Check sheet for the drawn part. Datum: minimum x, y, z corner. Units: mm. Give positions to 0.01 mm unless a question says otherwise; leave off trailing zeros. Loops run counter-clockwise (first coordinate to the right, second up) from the corner with the lowest first, then second, coordinate; pieces in that order, holes last.
1. Cross-section at A-A, the plane x = 16.5. Record the cut outline in (y, z).
2. Release check for a two-part mould opening along X. For the marked faces 1 and 2 record: +X half, -X half, draft (parallel to the pull), parting line (faces both ways), or undercut.
3. Cross-section at B-B, the plane z = 11.5. State how many separate pieces and enclosed holes the cut face has, plus the area to 3 significant figures.
4. Material ranges on L1, parallel to X at y = 0.15, z = 3; L2, parallel to Z at x = 19.5, y = 0.15 (1 decimal); L3, parallel to Z at x = 20, y = 0.5 (1 decimal), recorded low to high.
5. Go/stop test with flat-tipped pins: pin 1 Ø0.6 at (x, y) = (2.5, 0.5) entering from +Z; pin 2 Ø0.6 at (y, z) = (0.5, 3) entering from +X. Record where each tip stops, or that it passes through.
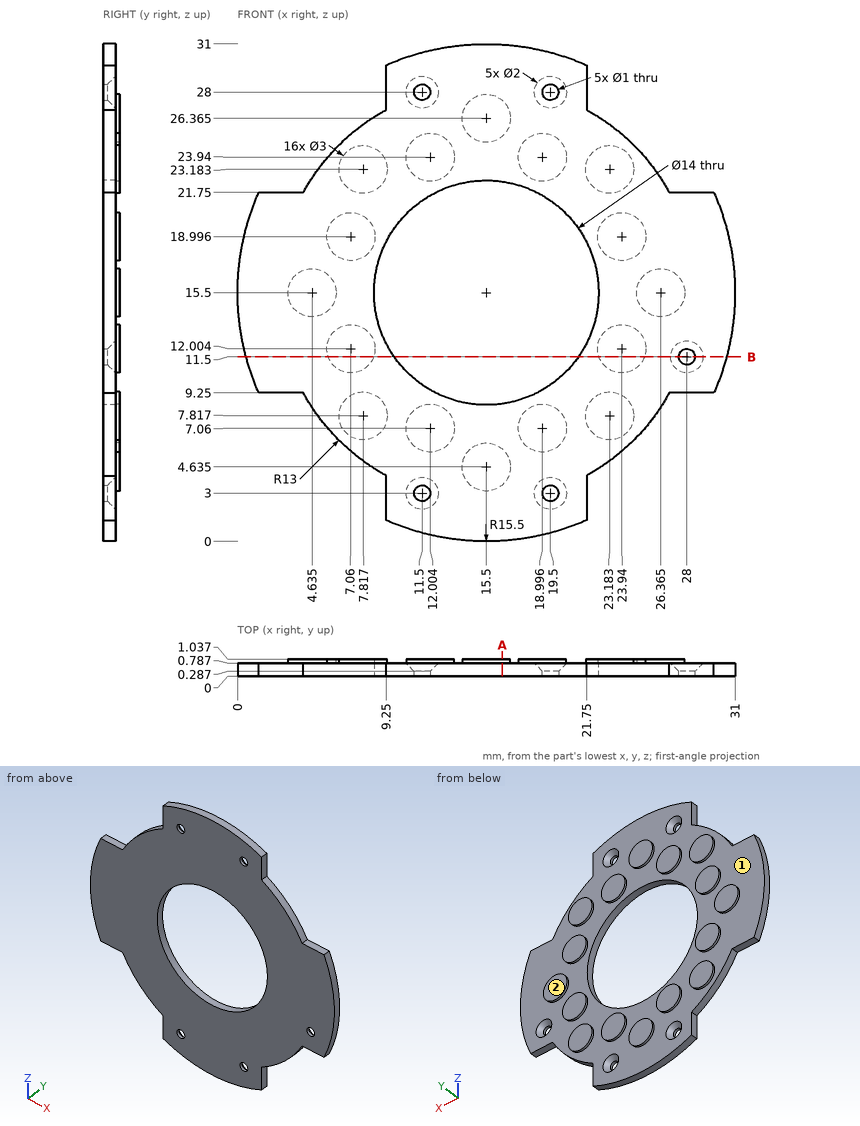
Result:
1. outline: (0, 0.03) - (0.79, 0.03) - (0.79, 3.52) - (1.04, 3.52) - (1.04, 5.75) - (0.79, 5.75) - (0.79, 8.57) - (0, 8.57) - close; (0, 22.43) - (0.79, 22.43) - (0.79, 25.25) - (1.04, 25.25) - (1.04, 27.48) - (0.79, 27.48) - (0.79, 30.97) - (0, 30.97) - close
2. face 1: undercut
2. face 2: draft
3. separate pieces: 3
3. enclosed holes: 0
3. area: 14.9 mm2
4. L1: x = 9.25 to 11, 12 to 19, 20 to 21.75
4. L2: z = 0.5 to 2.5, 3.5 to 9.8, 21.2 to 27.5, 28.5 to 30.5
4. L3: z = 0.7 to 2.5, 3.5 to 10.1, 20.9 to 27.5, 28.5 to 30.3
5. pin 1: stops at z = 21.75
5. pin 2: stops at x = 21.75
